Check sheet for the modelled part. Datum: model origin and axes. Units: mm. A direction names the side the tool comes from. Give positions to 0.01 mm unless a question says otherwise; leave off trailing zeros. Write each loop counter-clockwise with the first axis right and the second up, starting at its lowest first coordinate (ties: lowest second). Pieces come first, ordered by that corner, then holes. Notation, with made-up numbers: (-30.5, -35.5) -> (-7.5, -35.5) arc R29 cw to (-7.5, -1.5) -> close; hole circle Ø10 at (43, -38.5). An arc over 180 degrees is marked (long way). Answer as a JSON object with one key per item and string values.
Autodesk Inventor part; units mm, degrees
ref_plane "YZ Plane" through (0, 0, 0) normal (1, 0, 0) x (0, 1, 0)
ref_plane "XZ Plane" through (0, 0, 0) normal (0, 1, 0) x (-1, 0, 0)
ref_plane "XY Plane" through (0, 0, 0) normal (0, 0, 1) x (1, 0, 0)
sketch "Sketch1" plane through (0, 0, 0) normal (0, 0, 1) x (1, 0, 0)
  line L0 (0, 0) -> (0, 35)
  line L1 (0, 35) -> (5, 35)
  line L2 (5, 35) -> (5, 5)
  line L3 (5, 5) -> (63, 5)
  line L4 (63, 5) -> (63, 35)
  line L5 (63, 35) -> (68, 35)
  line L6 (68, 35) -> (68, 0)
  line L7 (68, 0) -> (0, 0)
  dimension "d0" = 35
  dimension "d1" = 5
  dimension "d2" = 30
  dimension "d3" = 58
  dimension "d4" = 30
  dimension "d5" = 5
extrude "Extrusion1" add sketch "Sketch1" along normal blind 30
sketch "Sketch2" plane through (68, 0, 0) normal (1, 0, 0) x (0, 0, -1)
  circle A0 centre (-15, 22.5) radius 5
  line L0 (0, 35) -> (-30, 35)
  line L1 (0, 0) -> (0, 35)
  dimension "d8" = 10
  dimension "d9" = 12.5
  dimension "d10" = 15
extrude "Extrusion2" cut sketch "Sketch2" against normal through all
sketch "Sketch3" plane through (5, 5, 0) normal (0, 1, 0) x (1, 0, 0)
  line L0 (15, -22.5) -> (43, -22.5)
  line L1 (43, -22.5) -> (43, -7.5)
  line L2 (43, -7.5) -> (15, -7.5)
  line L3 (15, -7.5) -> (15, -22.5)
  line L4 (15, -22.5) -> (43, -7.5) construction
  line L5 (43, -22.5) -> (15, -7.5) construction
  line L6 (58, 0) -> (0, 0)
  line L7 (0, 0) -> (0, -30)
  point P0 (-5, 0)
  point P1 (29, -15)
  dimension "d13" = 28
  dimension "d14" = 15
  dimension "d15" = 15
  dimension "d16" = 29
extrude "Extrusion3" cut sketch "Sketch3" against normal through all
sketch "Sketch4" plane through (5, 5, 0) normal (0, 1, 0) x (1, 0, 0)
  circle A0 centre (6, -14.0611) radius 3.625
  line L0 (0, -10) -> (0, -20)
  circle A1 centre (52, -14.0611) radius 3.625
  line L1 (43, -7.5) -> (43, -22.5)
  point P0 (-5, 0)
  dimension "d19" = 7.25
  dimension "d20" = 6
  dimension "d21" = 7.25
  dimension "d22" = 9
extrude "Extrusion4" cut sketch "Sketch4" against normal blind 2.1735 draft -45
sketch "Sketch5" plane through (11, 2.8265, 14.0611) normal (0, 1, 0) x (1, 0, 0)
  circle A0 centre (0, 0) radius 1.4515
  circle A1 centre (46, 0) radius 1.4515
  circle A2 centre (46, 0) radius 1.4515
  point P0 (-11, 14.0611)
extrude "Extrusion5" cut sketch "Sketch5" against normal through all
sketch "Sketch6" plane through (5, 5, 0) normal (0, 1, 0) x (1, 0, 0)
  point P0 (-5, 0)
properties part number "1st arm to 2nd linking clamp"
1. Access from +Z, -Z, +X, -X, +Y, -Y to the whole of each face (thin tool, end or side, straight path). Record for faces 1 (the face through (68, 18, 11)), 2 (the face through (34, 3, 22.5)), 3 (the face through (5, 17, 15)).
Determined:
{"face 1": "+Z, -Z, +X, +Y, -Y", "face 2": "+Y, -Y", "face 3": "+Z, -Z, +Y"}
2. Go/stop test with a flat-tipped pin: P1, Ø9, axis at x = 34.5, z = 20, coming from the +Y side. Record where the tip stops, or that it passes through.
Determined:
{"P1": "y = 5"}
3. Sectioned sample at D-D, the plane y = 22.5. Enter the section's corners in (x, z).
Determined:
{"outline": "(0, 0) -> (5, 0) -> (5, 10) -> (0, 10) -> close; (0, 20) -> (5, 20) -> (5, 30) -> (0, 30) -> close; (63, 0) -> (68, 0) -> (68, 10) -> (63, 10) -> close; (63, 20) -> (68, 20) -> (68, 30) -> (63, 30) -> close"}
4. Scan lines: L1, parallel to X at y = 18, z = 8; L2, parallel to Z at x = 11, y = 1.7; L3, parallel to X at y = 4.5, z = 18. Record each from-to range of solid material in increasing order. Write a range as [from, to].
Determined:
{"L1": "[0, 5], [63, 68]", "L2": "[0, 12.61], [15.51, 30]", "L3": "[0, 20], [48, 68]"}
5. Sectioned sample at A-A, the plane x = 41.5. Enter the section's corners in (y, z), plus the area to 3 significant figures.
Determined:
{"outline": "(0, 0) -> (5, 0) -> (5, 7.5) -> (0, 7.5) -> close; (0, 22.5) -> (5, 22.5) -> (5, 30) -> (0, 30) -> close", "area": "75.0 mm^2"}
6. Mould release check, pull along Y, two halves, no side actions. Record for faces 4 (the face through (2, 35, 15)), 5 (the face through (2.53, 17.62, 16.08)), 6 (the face through (36.4, 4.6, 0)): released by +Y, released by -Y, zero draft, split by the parting line, or undercut.
Determined:
{"face 4": "released by +Y", "face 5": "undercut", "face 6": "zero draft"}
7. Sectioned sample at C-C, the plane z = 6. Enter the section's corners in (x, y).
Determined:
{"outline": "(0, 0) -> (68, 0) -> (68, 35) -> (63, 35) -> (63, 5) -> (5, 5) -> (5, 35) -> (0, 35) -> close"}
8. Sectioned sample at B-B, the plane y = 31. Enter the section's corners in (x, z), plus the area to 3 significant figures.
Determined:
{"outline": "(0, 0) -> (5, 0) -> (5, 30) -> (0, 30) -> close; (63, 0) -> (68, 0) -> (68, 30) -> (63, 30) -> close", "area": "300 mm^2"}
